Check sheet for the modelled part. Datum: model origin and axes. Units: mm. A direction names the side the tool comes from. Coordinates: 2 decimals unless noted, no trailing zeros. Write each loop counter-clockwise with the first axis right and the second up, starting at its lowest first coordinate (ties: lowest second). Pieces come first, ordered by that corner, then holes. Notation, with made-up numbers: M 5.5,64.5 L 58.5,64.5 A22 ccw 58.5,100.5 Z; hole C 70.25,73.25 d3. An arc over 180 degrees is marked long. Answer as CSV lines item,"result".
Autodesk Inventor part; units mm, degrees
ref_plane "YZ Plane" through (0, 0, 0) normal (1, 0, 0) x (0, 1, 0)
ref_plane "XZ Plane" through (0, 0, 0) normal (0, 1, 0) x (-1, 0, 0)
ref_plane "XY Plane" through (0, 0, 0) normal (0, 0, 1) x (1, 0, 0)
sketch "Boceto1" plane through (0, 0, 0) normal (1, 0, 0) x (0, 1, 0)
  line L0 (-17, 17) -> (17, 17)
  line L1 (17, 17) -> (17, -17)
  line L2 (17, -17) -> (-17, -17)
  line L3 (-17, -17) -> (-17, 17)
  line L4 (-17, 17) -> (17, -17) construction
  line L5 (17, 17) -> (-17, -17) construction
  point P0 (0, 0)
  dimension "d0" = 34
  dimension "d1" = 34
extrude "Extrusión1" add sketch "Boceto1" along normal blind 1.5
sketch "Boceto2" plane through (0, 0, 0) normal (-1, 0, 0) x (0, 0, 1)
  line L0 (-20, -18.25) -> (20, -18.25)
  line L1 (20, -18.25) -> (20, 18.25)
  line L2 (20, 18.25) -> (-20, 18.25)
  line L3 (-20, 18.25) -> (-20, -18.25)
  line L4 (-20, -18.25) -> (20, 18.25) construction
  line L5 (20, -18.25) -> (-20, 18.25) construction
  point P0 (0, 0)
  dimension "d4" = 36.5
  dimension "d5" = 40
extrude "Extrusión2" add sketch "Boceto2" along normal blind 1.5
sketch "Boceto3" plane through (0, 0, 0) normal (1, 0, 0) x (0, 0, -1)
  line L0 (-20, 17.8927) -> (-20, -18.25)
  line L1 (-20, 18.25) -> (-20, -18.25)
  line L2 (20, -18.25) -> (-20, -18.25)
  line L3 (-18.15, -18.25) -> (-18.15, 18.25)
  line L4 (-18.15, 18.25) -> (-20, 18.25)
  line L5 (-20, -18.25) -> (-18.15, -18.25)
  line L6 (0, 18.25) -> (0, 10.0578) construction
  line L7 (20, 17.8927) -> (20, -18.25)
  line L8 (18.15, -18.25) -> (18.15, 18.25)
  line L9 (18.15, -18.25) -> (20, -18.25)
  point P0 (0, 0)
  dimension "d8" = 1.85
extrude "Extrusión3" add sketch "Boceto3" along normal blind 20
sketch "Boceto4" plane through (0, 0, 0) normal (1, 0, 0) x (0, 0, -1)
  line L0 (20, 18.25) -> (20, -18.25)
  line L1 (20, 18.25) -> (20, -18.25)
  line L2 (20, 18.25) -> (18.15, 18.25)
  line L3 (-18.15, 18.25) -> (20, 18.25)
  line L4 (18.15, 18.25) -> (18.15, -18.25)
  line L5 (18.15, -18.25) -> (20, -18.25)
  point P0 (0, 0)
  dimension "d11" = 1.85
extrude "Extrusión4" add sketch "Boceto4" along normal blind 20
sketch "Boceto5" plane through (-1.5, -18.25, 20) normal (0, 0, 1) x (1, 0, 0)
  line L0 (1.5, 18.25) -> (9.5, 18.25)
  line L1 (9.5, 18.25) -> (9.5, 30.25)
  line L2 (9.5, 18.25) -> (9.5, 6.25)
  dimension "d14" = 12
  dimension "d15" = 8
hole "Agujero1" at (8, 12, 20) at (8, -12, 20) direction (0, 0, -1) diameter 3 end through all
sketch "Boceto6" plane through (-1.5, 0, 0) normal (-1, 0, 0) x (0, 0, 1)
  line L0 (0, 0) -> (0, 8) construction
  circle A0 centre (0, 8) radius 1.1
  line L1 (0, 0) -> (7.3634, 0) construction
  circle A1 centre (0, -8) radius 1.1
  circle A2 centre (8, 8) radius 1.1
  circle A3 centre (8, -8) radius 1.1
  line L2 (0, 8) -> (-8, 8) construction
  circle A4 centre (-8, 8) radius 1.1
  circle A5 centre (-8, -8) radius 1.1
  line L3 (20, -18.25) -> (18.15, -18.25)
  line L4 (-20, 18.25) -> (-20, 9.1)
  dimension "d23" = 8
  dimension "d24" = 2.2
  dimension "d27" = 16
  dimension "d30" = 8
  dimension "d33" = 8
  dimension "d34" = 2.2
extrude "Extrusión5" cut sketch "Boceto6" against normal blind 10
properties part number "Tapa_R" material "Plástico ABS"
1) Section check D-D, the plane x = 8. Record the boundary of the cut face in (y, z), plus the area to 3 significant figures.
Answer key:
outline,"M -18.25,-20 L -13.5,-20 L -13.5,-18.15 L -18.25,-18.15 Z; M -18.25,18.15 L -13.5,18.15 L -13.5,20 L -18.25,20 Z; M -10.5,-20 L 10.5,-20 L 10.5,-18.15 L -10.5,-18.15 Z; M -10.5,18.15 L 10.5,18.15 L 10.5,20 L -10.5,20 Z; M 13.5,-20 L 18.25,-20 L 18.25,-18.15 L 13.5,-18.15 Z; M 13.5,18.15 L 18.25,18.15 L 18.25,20 L 13.5,20 Z"
area,"113 mm2"
2) Thickness scan on line 1 along Z through (x, y) = (0.25, -4.5); line 2 along Y through (x, z) = (0.95, -8); line 3 along Y through (x, z) = (-0.5, 0). Record the ranges inside material, lowest first.
Answer key:
line 1,"z = -20 to -18.15, -17 to 17, 18.15 to 20"
line 2,"y = -17 to -9.1, -6.9 to 6.9, 9.1 to 17"
line 3,"y = -18.25 to -9.1, -6.9 to 6.9, 9.1 to 18.25"
3) Section check B-B, the plane y = -8. Record the boundary of the cut face in (x, z), plus the area to 3 significant figures.
Answer key:
outline,"M -1.5,-20 L 20,-20 L 20,-18.15 L 0,-18.15 L 0,-17 L 1.5,-17 L 1.5,-9.1 L -1.5,-9.1 Z; M -1.5,-6.9 L 1.5,-6.9 L 1.5,-1.1 L -1.5,-1.1 Z; M -1.5,1.1 L 1.5,1.1 L 1.5,6.9 L -1.5,6.9 Z; M -1.5,9.1 L 1.5,9.1 L 1.5,17 L 0,17 L 0,18.15 L 20,18.15 L 20,20 L -1.5,20 Z"
area,"165 mm2"
4) Tool access check on faces 4 (the face through (1, 0, 17)), 5 (the face through (9.464, 12.325, -19.088)), 6 (the face through (1, -17, 0)), 7 (the face through (1, 17, 0)). Record the directions out of +Z, -Z, +X, -X, +Y, -Y that give a thin tool (end or side, any length) a straight path to the whole face; none if there is none.
Answer key:
face 4,"+X, +Y, -Y"
face 5,"+Z, -Z"
face 6,"+X, -Y"
face 7,"+X, +Y"
5) Mould release check, pull along Y, two halves, no side actions. Record for faces 1 (the face through (-0.4, -18.25, 1.6)), 2 (the face through (10, 0, 18.15)), 3 (the face through (-0.021, -9.074, -0.238)): pulls with the +Y half, pulls with the -Y half, needs draft (parallel to the pull), parting line crosses it, or undercut.
Answer key:
face 1,"pulls with the -Y half"
face 2,"needs draft"
face 3,"undercut"
6) Section check C-C, the plane z = 8. Record the boundary of the cut face in (x, y).
Answer key:
outline,"M -1.5,-18.25 L 0,-18.25 L 0,-17 L 1.5,-17 L 1.5,-9.1 L -1.5,-9.1 Z; M -1.5,-6.9 L 1.5,-6.9 L 1.5,6.9 L -1.5,6.9 Z; M -1.5,9.1 L 1.5,9.1 L 1.5,17 L 0,17 L 0,18.25 L -1.5,18.25 Z"
7) Depth check by flat-ended pin: P1, Ø1, axis at y = -14.5, z = 8, coming from the +X side; P2, Ø1.2, axis at x = 1, z = -4, coming from the +Y side. Enter the tip coordinate at first touch or a pass-through.
Answer key:
P1,"stops at x = 1.5"
P2,"stops at y = 17"
8) Section check A-A, the plane x = 2.25. Record the boundary of the cut face in (y, z), plus the area to 3 significant figures.
Answer key:
outline,"M -18.25,-20 L 18.25,-20 L 18.25,-18.15 L -18.25,-18.15 Z; M -18.25,18.15 L 18.25,18.15 L 18.25,20 L -18.25,20 Z"
area,"135 mm2"
